The model under review builds one solid part; all positions refer to its coordinate system, in mm. Face numbers are marked on the shaded views. A direction names the side the tool comes from. Coordinates: 2 decimals unless noted, no trailing zeros. Use CSV: the item, a comma, the result in double quotes. Start each with the question number.
from build123d import *

# Parameters (mm, degrees)
F0_W     = 55.5266755181
F0_H     = 46.0978470142
F1_DEPTH = 25.4


with BuildPart() as f1:
    # F0 (on Front) → F1 (new body)
    with BuildSketch(Plane.XZ):
        Polygon((-45.72, 27.7720657421), (-45.72, -27.7720657421), (45.72, -27.7720657421), (45.72, 2.3720657421), (45.72, 27.7720657421), align=None)
        with BuildLine():
            Line((45.72, 2.3720657421), (45.72, -27.7720657421))
            add(Edge.make_bspline(
                [(131.83991611, 27.7720657421), (128.4226083131, 3.6394915706), (87.0713041565, -12.0662870858), (45.72, -27.7720657421)],
                knots=[0.7528337274, 0.7528337274, 0.7528337274, 0.7528337274, 1, 1, 1, 1], degree=3))
            add(Edge.make_bspline(
                [(81.4163490426, 90.3064464871), (108.1552290461, 77.110332117), (134.8655063082, 49.1383822136), (131.83991611, 27.7720657421)],
                knots=[0.5339995176, 0.5339995176, 0.5339995176, 0.5339995176, 0.7528337274, 0.7528337274, 0.7528337274, 0.7528337274], degree=3))
            Line((81.4163490426, 90.3064464871), (104.9052251901, 53.874658511))
            ThreePointArc((104.9052251901, 53.874658511), (101.4010974206, 18.9161297578), (70.4063948109, 2.3720657421))
            Line((70.4063948109, 2.3720657421), (45.72, 2.3720657421))
        make_face()
        with BuildLine():
            add(Edge.make_bspline(
                [(131.83991611, 27.7720657421), (128.4226083131, 3.6394915706), (87.0713041565, -12.0662870858), (45.72, -27.7720657421)],
                knots=[0.7528337274, 0.7528337274, 0.7528337274, 0.7528337274, 1, 1, 1, 1], degree=3))
            add(Edge.make_bspline(
                [(45.72, -27.7720657421), (73.2817283043, -35.9046962959), (100.8434566087, -44.0373268496), (115.1341721416, -34.0887419879)],
                knots=[0, 0, 0, 0, 0.5105148873, 0.5105148873, 0.5105148873, 0.5105148873], degree=3))
            add(Edge.make_bspline(
                [(115.1341721416, -34.0887419879), (128.8362064561, -24.5499718093), (130.3380612831, 1.6110469664), (131.83991611, 27.7720657421)],
                knots=[0.5105148873, 0.5105148873, 0.5105148873, 0.5105148873, 1, 1, 1, 1], degree=3))
        make_face()
        with BuildLine():
            add(Edge.make_bspline(
                [(-45.72, 27.7720657421), (-25.4090292575, 29.6505869851), (-5.0980585151, 31.5291082281), (5.0941300286, 44.2085994729)],
                knots=[0, 0, 0, 0, 0.1784307554, 0.1784307554, 0.1784307554, 0.1784307554], degree=3))
            Line((-45.72, 27.7720657421), (45.72, 27.7720657421))
            Line((45.72, 27.7720657421), (70.4063948109, 27.7720657421))
            ThreePointArc((70.4063948109, 27.7720657421), (80.2980419597, 33.0519371353), (81.4163490426, 44.2085994729))
            Line((81.4163490426, 44.2085994729), (25.8896735245, 44.2085994729))
            Line((25.8896735245, 44.2085994729), (5.0941300286, 44.2085994729))
        make_face()
        with BuildLine():
            Line((45.72, 27.7720657421), (45.72, 2.3720657421))
            Line((45.72, 2.3720657421), (70.4063948109, 2.3720657421))
            ThreePointArc((70.4063948109, 2.3720657421), (101.4010974206, 18.9161297578), (104.9052251901, 53.874658511))
            Line((104.9052251901, 53.874658511), (81.4163490426, 44.2085994729))
            ThreePointArc((81.4163490426, 44.2085994729), (80.2980419597, 33.0519371353), (70.4063948109, 27.7720657421))
            Line((70.4063948109, 27.7720657421), (45.72, 27.7720657421))
        make_face()
        with BuildLine():
            add(Edge.make_bspline(
                [(5.0941300286, 44.2085994729), (15.012118023, 56.5469742394), (15.3484515231, 79.1129792412), (25.8896735245, 90.3064464871)],
                knots=[0.1784307554, 0.1784307554, 0.1784307554, 0.1784307554, 0.3520611864, 0.3520611864, 0.3520611864, 0.3520611864], degree=3))
            Line((5.0941300286, 44.2085994729), (25.8896735245, 44.2085994729))
            Line((25.8896735245, 44.2085994729), (25.8896735245, 90.3064464871))
        make_face()
        with Locations((53.6530112836, 67.25752298)):
            Rectangle(F0_W, F0_H)
        Polygon((104.9052251901, 53.874658511), (81.4163490426, 90.3064464871), (81.4163490426, 44.2085994729), align=None)
        with BuildLine():
            Line((25.8896735245, 90.3064464871), (81.4163490426, 90.3064464871))
            add(Edge.make_bspline(
                [(25.8896735245, 90.3064464871), (36.9352738157, 102.0355007707), (59.185696861, 101.2776699891), (81.4163490426, 90.3064464871)],
                knots=[0.3520611864, 0.3520611864, 0.3520611864, 0.3520611864, 0.5339995176, 0.5339995176, 0.5339995176, 0.5339995176], degree=3))
        make_face()
    extrude(amount=F1_DEPTH)


solid = f1.part
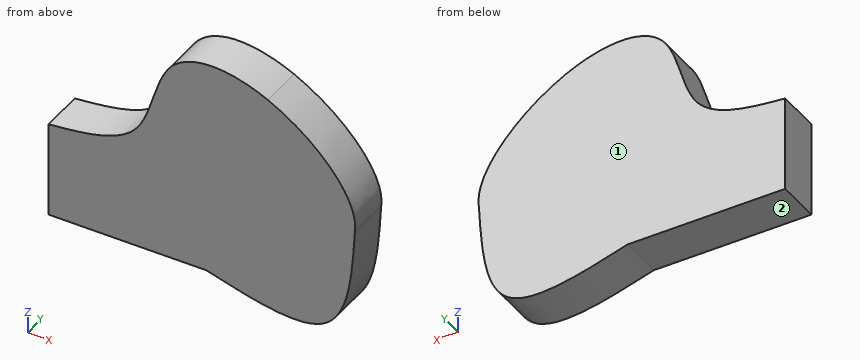
1. For the marked faces 1 and 2, list the 3-axis set-ups (+Z, -Z, +X, -X, +Y, -Y) from which the entire face can be reached by the end or side of a thin tool; tool diameter is ignored.
2. To check wall thickness, follow line 1 along Z through (x, y) = (88.5, -22.5); line 2 along Z through (x, y) = (73, -24.5); line 3 along X through (y, z) = (-23.25, 92). State the ranges of each line that lie inside material, in increasing order.
3. Insertion check: pin 1 Ø12 at (x, y) = (63, -8.5) entering from -Z; pin 2 Ø8 at (x, y) = (23, -4) entering from -Z; pin 3 Ø8 at (y, z) = (-11, 56.5) entering from +X. Each pin has a flat end and moves straight along its axis. Give the tip position at first contact, or say it passes through.
Solved:
1,face 1,"+Z, -Z, +X, -X, +Y"
1,face 2,"-Z, -X, +Y, -Y"
2,line 1,"z = -38.13 to 86.47"
2,line 2,"z = -35.28 to 93.98"
2,line 3,"x = 27.66 to 77.8"
3,pin 1,"stops at z = -34.31"
3,pin 2,"stops at z = -27.77"
3,pin 3,"stops at x = 124.88"
